```python
from build123d import *

# Parameters (mm, degrees)
SKETCH1_R             = 52.3875
SKETCH1_R_2           = 27.5
BOSS_EXTRUDE1_DEPTH   = 5.715
M6_CLEARANCE_HOLE1_D  = 6.6
F_5_0MM_DOWEL_HOLE1_D = 5
CIRPATTERN1_COUNT     = 4
CUT_EXTRUDE3_DEPTH    = 284.979078357
CUT_EXTRUDE4_DEPTH    = 284.979078357


with BuildPart() as part:
    # Sketch1 → Boss-Extrude1 (new, symmetric)
    with BuildSketch(Plane(origin=(0, 0, 0), x_dir=(1, 0, 0), z_dir=(0, 1, 0))):
        with BuildLine():
            Line((-62.780706514, -68.14502812), (-207.974881785, -9.956762437))
            ThreePointArc((-207.974881785, -9.956762437), (-218.225236723, -12.034965467), (-220.388836369, -22.267635732))
            Line((-220.388836369, -22.267635732), (-189.430137427, -101.422354045))
            ThreePointArc((-189.430137427, -101.422354045), (-188.283833694, -119.954004575), (-198.151371623, -135.681934472))
            Line((-198.151371623, -135.681934472), (-211.707233022, -147.086764223))
            ThreePointArc((-211.707233022, -147.086764223), (-214.295764489, -158.206433226), (-204.355245166, -163.82191268))
            Line((-204.355245166, -163.82191268), (-172.443362527, -159.700770109))
            ThreePointArc((-172.443362527, -159.700770109), (-168.164823601, -160.06920649), (-164.426538493, -162.182702446))
            ThreePointArc((-164.426538493, -162.182702446), (-143.500663309, -174.487669009), (-119.452254321, -177.801047868))
            Line((-119.452254321, -177.801047868), (57.036931174, -167.126674483))
            ThreePointArc((57.036931174, -167.126674483), (82.017871973, -156.408307566), (94.466622628, -132.24305566))
            Line((94.466622628, -132.24305566), (108.629935196, -24.576488538))
            ThreePointArc((108.629935196, -24.576488538), (102.609116202, -14.445444869), (91.348434445, -17.92184438))
            Line((91.348434445, -17.92184438), (65.060480918, -55.990558325))
            ThreePointArc((65.060480918, -55.990558325), (54.61, -61.474087679), (44.159519082, -55.990558325))
            Line((44.159519082, -55.990558325), (17.871565555, -17.92184438))
            ThreePointArc((17.871565555, -17.92184438), (9.247910088, -13.841666007), (1.412558245, -19.284326264))
            Line((1.412558245, -19.284326264), (-12.176603989, -48.212200061))
            ThreePointArc((-12.176603989, -48.212200061), (-33.518744337, -68.231765471), (-62.780706514, -68.14502812))
        make_face()
        with Locations(Location((-123.19, -116.001477372, 0), (0, 0, 270))):
            Circle(SKETCH1_R, mode=Mode.SUBTRACT)
        with Locations(Location((54.61, -127, 0), (0, 0, 270))):
            Circle(SKETCH1_R_2, mode=Mode.SUBTRACT)
    extrude(amount=BOSS_EXTRUDE1_DEPTH, both=True)

    # M6 Clearance Hole1 (through all)
    with Locations(Plane(origin=(0, -5.715, 0), x_dir=(-1, 0, 0), z_dir=(0, -1, 0))):
        with Locations((-222.084502927, -125.821700696), (-10.033704867, -23.334197365), (-99.186295133, -23.334197365), (211.518182886, -18.798178744), (205.575185514, -154.375359311)):
            Hole(M6_CLEARANCE_HOLE1_D / 2)

    # Ø5.0mm Dowel Hole1 (through all)
    with Locations(Plane(origin=(0, 5.715, 0), x_dir=(1, 0, 0), z_dir=(0, 1, 0))):
        with Locations((-123.19, -173.151477372)):
            f_5_0mm_dowel_hole1 = Hole(F_5_0MM_DOWEL_HOLE1_D / 2)

    # CirPattern1: Ø5.0mm Dowel Hole1 ×4 about axis
    cirpattern1_axis = Axis((-123.19, 0, 116.001477372), (0, 1, 0))
    for i in range(1, CIRPATTERN1_COUNT):
        add(f_5_0mm_dowel_hole1.rotate(cirpattern1_axis, i * 360 / CIRPATTERN1_COUNT), mode=Mode.SUBTRACT)

    # Sketch12 → Cut-Extrude3 (cut, through all)
    with BuildSketch(Plane.XZ.offset(5.715)):
        with BuildLine():
            Line((-14.234653979, 76.580666612), (2.016277078, 40.924992231))
            ThreePointArc((2.016277078, 40.924992231), (11.084872861, 34.469497273), (21.201297863, 39.113933708))
            Line((21.201297863, 39.113933708), (46.984841737, 75.545913676))
            ThreePointArc((46.984841737, 75.545913676), (47.441443369, 82.132150292), (41.801580719, 85.564197365))
            Line((41.801580719, 85.564197365), (-8.456504121, 85.564197365))
            ThreePointArc((-8.456504121, 85.564197365), (-13.797169823, 82.649279585), (-14.234653979, 76.580666612))
        make_face()
        with BuildLine():
            Line((-204.660650751, 36.331409888), (-188.626913597, 77.326218823))
            ThreePointArc((-188.626913597, 77.326218823), (-183.343464985, 81.400582198), (-177.265672517, 78.648182362))
            ThreePointArc((-177.265672517, 78.648182362), (-164.864290964, 65.181201114), (-149.229324423, 55.657458697))
            ThreePointArc((-149.229324423, 55.657458697), (-145.319075006, 49.625624375), (-149.386073966, 43.698348841))
            Line((-149.386073966, 43.698348841), (-194.042740287, 25.801666969))
            ThreePointArc((-194.042740287, 25.801666969), (-202.810079512, 27.579196728), (-204.660650751, 36.331409888))
        make_face()
        with BuildLine():
            Line((-190.985681304, 136.027573744), (-194.692687992, 140.689511725))
            ThreePointArc((-194.692687992, 140.689511725), (-195.773357295, 149.809803058), (-188.096484537, 154.850952212))
            Line((-188.096484537, 154.850952212), (-182.142551509, 155.01295786))
            ThreePointArc((-182.142551509, 155.01295786), (-179.298484939, 153.425933155), (-179.332786017, 150.169219243))
            ThreePointArc((-179.332786017, 150.169219243), (-182.766707481, 143.751485155), (-185.46990532, 136.993390091))
            ThreePointArc((-185.46990532, 136.993390091), (-187.940827525, 134.871620657), (-190.985681304, 136.027573744))
        make_face()
    extrude(amount=-CUT_EXTRUDE3_DEPTH, mode=Mode.SUBTRACT)

    # Sketch13 → Cut-Extrude4 (cut, through all)
    with BuildSketch(Plane.XZ.offset(5.715)):
        with BuildLine():
            Line((7.636577505, 114.096477372), (-48.751422495, 114.096477372))
            ThreePointArc((-48.751422495, 114.096477372), (-58.276422495, 104.571477372), (-48.751422495, 95.046477372))
            Line((-48.751422495, 95.046477372), (7.636577505, 95.046477372))
            ThreePointArc((7.636577505, 95.046477372), (17.161577505, 104.571477372), (7.636577505, 114.096477372))
        make_face()
        with BuildLine():
            ThreePointArc((-59.54342217, 132.642118181), (-56.149544678, 127.512420027), (-50.328184067, 125.526477372))
            Line((-50.328184067, 125.526477372), (2.447685954, 125.526477372))
            ThreePointArc((2.447685954, 125.526477372), (16.711385269, 138.163192745), (4.074669896, 152.42689206))
            Line((4.074669896, 152.42689206), (-58.528880044, 156.213263816))
            Line((-58.528880044, 156.213263816), (-59.309504972, 156.260477372))
            ThreePointArc((-59.309504972, 156.260477372), (-64.85762699, 153.125613078), (-65.035173244, 146.755565245))
            ThreePointArc((-65.035173244, 146.755565245), (-61.881820392, 139.857397165), (-59.54342217, 132.642118181))
        make_face()
    extrude(amount=-CUT_EXTRUDE4_DEPTH, mode=Mode.SUBTRACT)


solid = part.part
```
Source: CAD feature listing. Evaluate the final solid. Frame: model axes, mm. A direction names the side the tool comes from. Round coordinates to 2 decimals unless told otherwise and drop trailing zeros. Loops run counter-clockwise (first coordinate to the right, second up) from the corner with the lowest first, then second, coordinate; pieces in that order, holes last. Notation, with made-up numbers: M 39,-3.75 L 73,-3.75 A11 ccw 73,8.25 Z; hole C 10.25,88.5 d7. An arc over 180 degrees is marked long. Use a Markdown table: item, result. Add a question column.
1. Contact query for flat-ended pins moving along their axis: P1, Ø5.5, axis at x = -205.58, z = 154.38, coming from the +Y side; P2, Ø3, axis at x = -185, y = -3, coming from the -Z side; P3, Ø2, axis at y = -3.5, z = 47, coming from the +X side; P4, Ø5.5, axis at x = -11.5, y = 2.5, coming from the +Z side. Output: stop coordinate, or through.
2. Mould query, pull axis Z, two halves, no side actions, for faces 4 (the cylindrical face through (-33.129, 0.08, 68.076)), 5 (the cylindrical face through (10.922, -0.08, 34.486)), 6 (the cylindrical face through (-143.823, 0.08, 174.375)), 7 (the cylindrical face through (102.334, 0.08, 22.343)). Classes: pulls with the +Z half, pulls with the -Z half, needs draft (parallel to the pull), parting line crosses it, or undercut.
3. Section query B-B on x = -83.5. Return the cut outline in (y, z) (3 decimals), then the cut area to 3 significant figures.
4. Section query A-A on x = -27. Return the cut outline in (y, z) (3 decimals).
5. Line query: line 1 (X direction, y = 1, z = 84); line 2 (Z direction, x = -26.5, y = 0.5); line 3 (X direction, y = 2.75, z = 127). Output: solid intervals per line, ascending.
6. Section query C-C on y = -3.25. Give the number of separate pieces and of enclosed holes in the cut face, then the cut area to 3 significant figures.
7. Reachability of faces 1 (the cylindrical face through (81.7, 0.1, 156.7)), 2 (the cylindrical face through (-165.06, -0.08, 65.34)), 3 (the flat face through (-204.83, 0.08, 141.3)) from +Z, -Z, +X, -X, +Y, -Y: full face, straight path, thin tool, end or side. Return the list, or none.
Reported:
| question | item | result |
|---|---|---|
| 1 | P1 | passes through |
| 1 | P2 | stops at z = 18.56 |
| 1 | P3 | stops at x = 105.81 |
| 1 | P4 | stops at z = 171.44 |
| 2 | face 4 | pulls with the -Z half |
| 2 | face 5 | undercut |
| 2 | face 6 | pulls with the +Z half |
| 2 | face 7 | undercut |
| 3 | outline | M -5.715,59.842 L 5.715,59.842 L 5.715,81.809 L -5.715,81.809 Z; M -5.715,150.194 L 5.715,150.194 L 5.715,175.627 L -5.715,175.627 Z |
| 3 | area | 542 mm² |
| 4 | outline | M -5.715,64.941 L 5.715,64.941 L 5.715,95.046 L -5.715,95.046 Z; M -5.715,114.096 L 5.715,114.096 L 5.715,125.526 L -5.715,125.526 Z; M -5.715,154.306 L 5.715,154.306 L 5.715,172.209 L -5.715,172.209 Z |
| 5 | line 1 | x = -196.24 to -164.67, -81.71 to -12.63, 45.98 to 100.81 |
| 5 | line 2 | z = 64.62 to 95.05, 114.1 to 125.53, 154.28 to 172.18 |
| 5 | line 3 | x = -191.05 to -174.41, -71.97 to -55.42, 9.44 to 27.11, 82.11 to 95.16 |
| 6 | separate pieces | 1 |
| 6 | enclosed holes | 15 |
| 6 | area | 19,500 mm² |
| 7 | face 1 | +Z, +X, +Y, -Y |
| 7 | face 2 | +Y, -Y |
| 7 | face 3 | -X, +Y, -Y |
